from build123d import *

# Parameters (mm, degrees)
SKETCH1_R               = 2.1
SKETCH1_R_2             = 10
BOSS_EXTRUDE1_DEPTH     = 3
SKETCH2_W               = 88
SKETCH2_H               = 4
CUT_EXTRUDE1_DEPTH      = 1
CUT_EXTRUDE1_DEPTH_BACK = 4


with BuildPart() as part:
    # Sketch1 → Boss-Extrude1 (new body)
    with BuildSketch(Plane(origin=(0, 0, 0), x_dir=(1, 0, 0), z_dir=(0, 1, 0))):
        with BuildLine():
            Line((-8, 26), (-8, 66))
            ThreePointArc((-8, 66), (-9.757359313, 70.242640687), (-14, 72))
            Line((-14, 72), (-24, 72))
            Line((-24, 72), (-24, 135))
            ThreePointArc((-24, 135), (-25.757359313, 139.242640687), (-30, 141))
            Line((-30, 141), (-58, 141))
            ThreePointArc((-58, 141), (-62.242640687, 139.242640687), (-64, 135))
            Line((-64, 135), (-64, -43))
            Line((-64, -43), (-24, -43))
            Line((-24, -43), (24, -43))
            Line((24, -43), (24, 24))
            Line((24, 24), (-6, 24))
            ThreePointArc((-6, 24), (-7.414213562, 24.585786438), (-8, 26))
        make_face()
        with Locations((16, 16)):
            Circle(SKETCH1_R, mode=Mode.SUBTRACT)
        with Locations((16, -16)):
            Circle(SKETCH1_R, mode=Mode.SUBTRACT)
        with Locations((-16, -16)):
            Circle(SKETCH1_R, mode=Mode.SUBTRACT)
        with Locations((-16, 16)):
            Circle(SKETCH1_R, mode=Mode.SUBTRACT)
        with Locations((-16, 32)):
            Circle(SKETCH1_R, mode=Mode.SUBTRACT)
        with Locations((-16, 64)):
            Circle(SKETCH1_R, mode=Mode.SUBTRACT)
        with Locations((-44, 0)):
            Circle(SKETCH1_R_2, mode=Mode.SUBTRACT)
        with Locations((-44, 35)):
            Circle(SKETCH1_R_2, mode=Mode.SUBTRACT)
        with Locations((-44, 70)):
            Circle(SKETCH1_R_2, mode=Mode.SUBTRACT)
        with Locations((-44, 105)):
            Circle(SKETCH1_R_2, mode=Mode.SUBTRACT)
    extrude(amount=BOSS_EXTRUDE1_DEPTH)

    # Sketch2 → Cut-Extrude1 (cut, two sides)
    with BuildSketch(Plane(origin=(0, 3, 0), x_dir=(1, 0, 0), z_dir=(0, 1, 0))) as cut_extrude1_sk:
        with Locations((-20, -41)):
            Rectangle(SKETCH2_W, SKETCH2_H)
    extrude(amount=CUT_EXTRUDE1_DEPTH, mode=Mode.SUBTRACT)
    extrude(cut_extrude1_sk.sketch, amount=-CUT_EXTRUDE1_DEPTH_BACK, mode=Mode.SUBTRACT)


solid = part.part
Can you work these out from the model? Positions are in its coordinate system, mm. Give positions to 0.01 mm unless a question says otherwise; leave off trailing zeros. Loops run counter-clockwise (first coordinate to the right, second up) from the corner with the lowest first, then second, coordinate; pieces in that order, holes last. Notation, with made-up numbers: (-38, 58) - (-6, 58) arc R13 cw to (-6, 79) - close; hole circle Ø2 at (-33.75, -19). An arc over 180 degrees is marked (long way). Answer as a JSON object with one key per item and string values.
Q1. Imagine slicing it at C-C on x = -16. Write out the boundary of the cut face in (y, z).
Geometry says:
{"outline": "(0, -72) - (3, -72) - (3, -66.1) - (0, -66.1) - close; (0, -61.9) - (3, -61.9) - (3, -34.1) - (0, -34.1) - close; (0, -29.9) - (3, -29.9) - (3, -18.1) - (0, -18.1) - close; (0, -13.9) - (3, -13.9) - (3, 13.9) - (0, 13.9) - close; (0, 18.1) - (3, 18.1) - (3, 39) - (0, 39) - close"}
Q2. Imagine slicing it at B-B on y = 2.55. Give the number of separate pieces and of enclosed holes in the cut face, plus the area to 3 significant figures.
Geometry says:
{"separate pieces": "1", "enclosed holes": "10", "area": "9,630 mm²"}
Q3. Imagine slicing it at A-A on z = -105. Write out the boundary of the cut face in (x, y).
Geometry says:
{"outline": "(-64, 0) - (-54, 0) - (-54, 3) - (-64, 3) - close; (-34, 0) - (-24, 0) - (-24, 3) - (-34, 3) - close"}
Q4. Imagine slicing it at D-D on z = -64. Write out the boundary of the cut face in (x, y), plus the area to 3 significant figures.
Geometry says:
{"outline": "(-64, 0) - (-52, 0) - (-52, 3) - (-64, 3) - close; (-36, 0) - (-18.1, 0) - (-18.1, 3) - (-36, 3) - close; (-13.9, 0) - (-8, 0) - (-8, 3) - (-13.9, 3) - close", "area": "107 mm²"}
Q5. Will these pins go through, and if not, where does the flat tip stop? P1, Ø0.9, axis at x = -18.5, y = 1.5, coming from the -Z side; P2, Ø1.5, axis at y = 1.5, z = -44, coming from the +X side.
Geometry says:
{"P1": "z = -72", "P2": "x = -8"}
Q6. If we mould it in two halves opening along X, with no side actions, what happens to faces 1 (the flat face through (-30, 3, -32)), 2 (the cylindrical face through (15.727, 1.479, 13.918)), 3 (the cylindrical face through (-25.711, 1.479, -139.196)), 4 (the cylindrical face through (-46.17, 1.48, -25.24))? For each: pulls with the +X half, pulls with the -X half, needs draft (parallel to the pull), parting line crosses it, or undercut.
Geometry says:
{"face 1": "needs draft", "face 2": "undercut", "face 3": "pulls with the +X half", "face 4": "undercut"}
Q7. If I drill on L1, parallel to X at y = 1.8, z = -16; L2, parallel to Z at x = -16, y = 1.5; L3, parallel to Z at x = -44, y = 1.75, over which ranges is the centre line in solid material (lowest first)?
Geometry says:
{"L1": "-64 to -18.1, -13.9 to 13.9, 18.1 to 24", "L2": "-72 to -66.1, -61.9 to -34.1, -29.9 to -18.1, -13.9 to 13.9, 18.1 to 39", "L3": "-141 to -115, -95 to -80, -60 to -45, -25 to -10, 10 to 39"}
